Geometry: final body of the model. Coordinates: model frame, mm. A direction names the side the tool comes from. Round coordinates to 2 decimals unless told otherwise and drop trailing zeros. Loops run counter-clockwise (first coordinate to the right, second up) from the corner with the lowest first, then second, coordinate; pieces in that order, holes last. Notation, with made-up numbers: (-27, 57) - (9, 57) arc R15 cw to (9, 84) - close; hole circle Ø9 at (-7, 2.25). An arc over 180 degrees is marked (long way). Return JSON: item names as keys, results as strings. Group by question number.
1. Section C-C on z = 36.5. Return loops of the section in (x, y), and give its area (3 significant figures).
2. Section A-A on y = -100. Return loops of the section in (x, z).
3. Material intervals for probe 1 along Y at (x, z) = (45.39, 95.25); probe 2 along X at (y, z) = (-70.5, 88); probe 3 along Z at (x, y) = (-45.39, -3), sorted ascending.
4. Draft query along Y for faces 6 (the face through (1.22, -3.82, -96.38)), 7 (the face through (-93.74, -43.55, 56.72)), 8 (the face through (-14.985, -193.739, 0.66)). Return one class per face: +Y half, -Y half, draft (parallel to the pull), parting line (faces both ways), or undercut.
5. First-contact query: pin 1 Ø24 at (x, y) = (45.39, -146.58) entering from -Z; pin 2 Ø15 at (y, z) = (-101, 0) entering from +X; pin 3 Ø10 at (x, z) = (48.5, 43) entering from +Y. Flat tips, straight axial feed; report the tip coordinate or a pass-through.
6. Set-up query: faces 1 (the face through (87.3, -146, 47)), 2 (the face through (42.14, -68.06, 93.74)), 3 (the face through (-47.343, -161.456, -93.739)), 4 (the face through (0, -187.3, 0)), 5 (the face through (-46, -12.7, 47)). Return all of +Z, -Z, +X, -X, +Y, -Y with unobstructed straight access to the full face (end or side cutting, diameter ignored); none if empty.
7. Section B-B on x = 0. Return loops of the section in (y, z), and give its area (3 significant figures).
from build123d import *

# Parameters (mm, degrees)
F0_W      = 200
F0_H      = 200
F1_DEPTH  = 200
F2_R      = 12.7
F3_R      = 15
F4_DEPTH  = 12.7
F5_R      = 15
F6_DEPTH  = 12.7
F7_R      = 15
F8_DEPTH  = 12.7
F9_R      = 15
F10_DEPTH = 12.7
F11_R     = 15
F12_DEPTH = 12.7
F13_R     = 15
F14_DEPTH = 12.7


with BuildPart() as f1:
    # F0 (on Front) → F1 (new body)
    with BuildSketch(Plane.XZ):
        Rectangle(F0_W, F0_H)
    extrude(amount=F1_DEPTH)

    # F2
    f2_edges = [f1.edges().sort_by_distance(p)[0] for p in [
        (0, -200, 100),
        (100, -100, 100),
        (-100, -100, 100),
        (-100, -200, 0),
        (0, -200, -100),
        (100, -200, 0),
        (-100, -100, -100),
        (0, 0, 100),
        (-100, 0, 0),
        (0, 0, -100),
        (100, -100, -100),
        (100, 0, 0),
    ]]
    fillet(f2_edges, radius=F2_R)

    # F3 (on face) → F4 (cut)
    with BuildSketch(Plane.XZ.offset(200)):
        Circle(F3_R)
    extrude(amount=-F4_DEPTH, mode=Mode.SUBTRACT)

    # F5 (on face) → F6 (cut)
    with BuildSketch(Plane(origin=(-100, 0, 0), x_dir=(0, -1, 0), z_dir=(-1, 0, 0))):
        with Locations((54.61, 46.586072)):
            Circle(F5_R)
        with Locations((145.39, -46.5838)):
            Circle(F5_R)
    extrude(amount=-F6_DEPTH, mode=Mode.SUBTRACT)

    # F7 (on face) → F8 (cut)
    with BuildSketch(Plane.YZ.offset(100)):
        with Locations((-145.39, 46.5838)):
            Circle(F7_R)
        with Locations((-100, 0)):
            Circle(F7_R)
        with Locations((-54.61, -46.5838)):
            Circle(F7_R)
    extrude(amount=-F8_DEPTH, mode=Mode.SUBTRACT)

    # F9 (on face) → F10 (cut)
    with BuildSketch(Plane.XZ):
        with Locations((45.39, 46.5838)):
            Circle(F9_R)
        with Locations((45.39, -46.5838)):
            Circle(F9_R)
        with Locations((-45.39, -46.5838)):
            Circle(F9_R)
        with Locations((-45.39, 46.5838)):
            Circle(F9_R)
    extrude(amount=F10_DEPTH, mode=Mode.SUBTRACT)

    # F11 (on face) → F12 (cut)
    with BuildSketch(Plane.XY.offset(100)):
        with Locations((0, -100)):
            Circle(F11_R)
        with Locations((-45.39, -53.4162)):
            Circle(F11_R)
        with Locations((45.39, -53.4162)):
            Circle(F11_R)
        with Locations((-45.39, -146.5838)):
            Circle(F11_R)
        with Locations((45.39, -146.5838)):
            Circle(F11_R)
    extrude(amount=-F12_DEPTH, mode=Mode.SUBTRACT)

    # F13 (on face) → F14 (cut)
    with BuildSketch(Plane(origin=(0, 0, -100), x_dir=(1, 0, 0), z_dir=(0, 0, -1))):
        with Locations((45.39, 53.4162)):
            Circle(F13_R)
        with Locations((45.39, 100)):
            Circle(F13_R)
        with Locations((45.39, 146.5838)):
            Circle(F13_R)
        with Locations((-45.39, 53.4162)):
            Circle(F13_R)
        with Locations((-45.39, 100)):
            Circle(F13_R)
        with Locations((-45.39, 146.5838)):
            Circle(F13_R)
    extrude(amount=-F14_DEPTH, mode=Mode.SUBTRACT)


solid = f1.part
Taken from the geometry:
{
 "1": {"outline": "(-100, -187.3) arc R12.7 ccw to (-87.3, -200) - (87.3, -200) arc R12.7 ccw to (100, -187.3) - (100, -156.49) - (87.3, -156.49) - (87.3, -134.29) - (100, -134.29) - (100, -12.7) arc R12.7 ccw to (87.3, 0) - (56.49, 0) - (56.49, -12.7) - (34.29, -12.7) - (34.29, 0) - (-34.29, 0) - (-34.29, -12.7) - (-56.49, -12.7) - (-56.49, 0) - (-87.3, 0) arc R12.7 ccw to (-100, -12.7) - (-100, -43.51) - (-87.3, -43.51) - (-87.3, -65.71) - (-100, -65.71) - close", "area": "38,700 mm2"},
 "2": {"outline": "(-100, -87.3) arc R12.7 ccw to (-87.3, -100) - (-60.39, -100) - (-60.39, -87.3) - (-30.39, -87.3) - (-30.39, -100) - (30.39, -100) - (30.39, -87.3) - (60.39, -87.3) - (60.39, -100) - (87.3, -100) arc R12.7 ccw to (100, -87.3) - (100, -15) - (87.3, -15) - (87.3, 15) - (100, 15) - (100, 87.3) arc R12.7 ccw to (87.3, 100) - (15, 100) - (15, 87.3) - (-15, 87.3) - (-15, 100) - (-87.3, 100) arc R12.7 ccw to (-100, 87.3) - close"},
 "3": {"probe 1": "-197.2 to -161.58, -131.58 to -68.42, -38.42 to -2.8", "probe 2": "-99.98 to 99.98", "probe 3": "-95.5 to -61.58, -31.58 to 31.58, 61.58 to 95.5"},
 "4": {"face 6": "+Y half", "face 7": "undercut", "face 8": "draft"},
 "5": {"pin 1": "z = -87.3", "pin 2": "x = 87.3", "pin 3": "y = -12.7"},
 "6": {"face 1": "+X", "face 2": "+Z", "face 3": "-Z", "face 4": "-Y", "face 5": "+Y"},
 "7": {"outline": "(-200, -87.3) arc R12.7 ccw to (-187.3, -100) - (-12.7, -100) arc R12.7 ccw to (0, -87.3) - (0, 87.3) arc R12.7 ccw to (-12.7, 100) - (-85, 100) - (-85, 87.3) - (-115, 87.3) - (-115, 100) - (-187.3, 100) arc R12.7 ccw to (-200, 87.3) - (-200, 15) - (-187.3, 15) - (-187.3, -15) - (-200, -15) - close", "area": "39,100 mm2"}
}
